```python
from build123d import *

# Parameters (mm, degrees)
SKETCH1_W           = 17.9
SKETCH1_H           = 14
BOSS_EXTRUDE1_DEPTH = 6
SKETCH2_R           = 1.75
CUT_EXTRUDE1_DEPTH  = 15
CUT_EXTRUDE2_DEPTH  = 6
CHAMFER1_SIZE       = 0.25


with BuildPart() as part:
    # Sketch1 → Boss-Extrude1 (new body)
    with BuildSketch(Plane.XY):
        with Locations((0, 7)):
            Rectangle(SKETCH1_W, SKETCH1_H)
    extrude(amount=BOSS_EXTRUDE1_DEPTH)

    # Sketch2 → Cut-Extrude1 (cut, through all)
    with BuildSketch(Plane(origin=(0, 14, 0), x_dir=(1, 0, 0), z_dir=(0, 1, 0))):
        with Locations((0, -3)):
            Circle(SKETCH2_R)
    extrude(amount=-CUT_EXTRUDE1_DEPTH, mode=Mode.SUBTRACT)

    # Sketch3 → Cut-Extrude2 (cut)
    with BuildSketch(Plane.XY.offset(6)):
        Polygon((5, 14), (5, 2), (5.7, 2), (5.7, 2.2), (6.6, 3.1), (5.7, 4), (5.7, 4.2), (6.6, 5.1), (5.7, 6), (5.7, 6.2), (6.6, 7.1), (5.7, 8), (5.7, 8.2), (6.6, 9.1), (5.7, 10), (5.7, 10.2), (6.6, 11.1), (5.7, 12), (5.7, 12.2), (6.6, 13.1), (5.7, 14), align=None)
        Polygon((-5.7, 2.2), (-5.7, 2), (-5, 2), (-5, 14), (-5.7, 14), (-6.6, 13.1), (-5.7, 12.2), (-5.7, 12), (-6.6, 11.1), (-5.7, 10.2), (-5.7, 10), (-6.6, 9.1), (-5.7, 8.2), (-5.7, 8), (-6.6, 7.1), (-5.7, 6.2), (-5.7, 6), (-6.6, 5.1), (-5.7, 4.2), (-5.7, 4), (-6.6, 3.1), align=None)
    extrude(amount=-CUT_EXTRUDE2_DEPTH, mode=Mode.SUBTRACT)

    # Chamfer1
    chamfer1_edges = [part.edges().sort_by_distance(p)[0] for p in [
        (8.95, 7, 6),
        (0, 14, 0),
        (-7.325, 14, 0),
        (-8.95, 7, 6),
        (7.325, 14, 0),
        (8.95, 7, 0),
        (0, 0, 0),
        (-8.95, 7, 0),
        (0, 0, 6),
    ]]
    chamfer(chamfer1_edges, length=CHAMFER1_SIZE)


solid = part.part
```
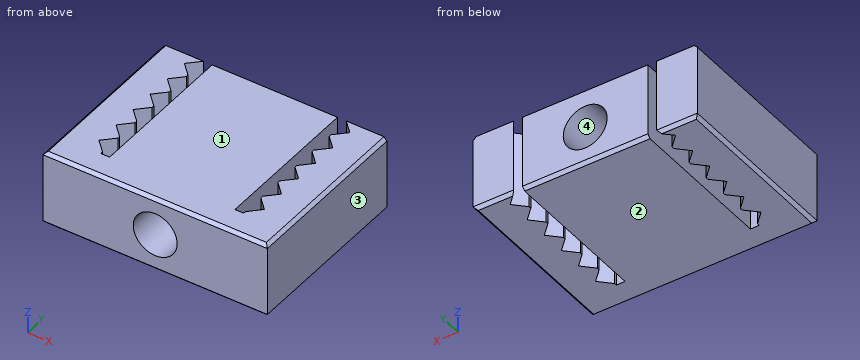
Input: part model. Units: mm. Frame: model coordinates. Face numbers are marked on the shaded views. Round coordinates to 2 decimals unless told otherwise and drop trailing zeros. Write each loop counter-clockwise with the first axis right and the second up, starting at its lowest first coordinate (ties: lowest second). Pieces come first, ordered by that corner, then holes. Notation, with made-up numbers: M 84.5,54.5 L 131.5,54.5 A15 cw 131.5,74.5 Z; hole C 68.5,1 d4. An arc over 180 degrees is marked long. Write each question's results on one line, items separated by ' | '.
Q1. Draft query along Z for the marked faces 1, 2, 3 and 4. Return one class per face: released by +Z, released by -Z, zero draft, split by the parting line, or undercut.
Results:
face 1: released by +Z | face 2: released by -Z | face 3: zero draft | face 4: undercut
Q2. Pin query (flat end, axial travel): P1, Ø2, axis at x = 0, z = 3, coming from the -Y side. Return the tip coordinate at first contact, or that it passes through.
Results:
P1: passes through
Q3. Section query A-A (y = 7.5). Return loops of the section in (x, z).
Results:
outline: M -8.95,0.25 L -8.7,0 L -6.2,0 L -6.2,6 L -8.7,6 L -8.95,5.75 Z; M -5,0 L 5,0 L 5,6 L -5,6 Z; M 6.2,0 L 8.7,0 L 8.95,0.25 L 8.95,5.75 L 8.7,6 L 6.2,6 Z; hole C 0,3 d3.5
Q4. Section query B-B (x = 0). Return loops of the section in (y, z), and give its area (3 significant figures).
Results:
outline: M 0,0.25 L 0.25,0 L 13.75,0 L 14,0.25 L 14,1.25 L 0,1.25 Z; M 0,4.75 L 14,4.75 L 14,6 L 0.25,6 L 0,5.75 Z | area: 34.9 mm^2
Q5. Line query: line 1 along X through (y, z) = (6.5, 2.25); line 2 along X through (y, z) = (9.5, 3); line 3 along X through (y, z) = (11.5, 0.75). Output: solid intervals per line, ascending.
Results:
line 1: x = -8.95 to -6, -5 to -1.58, 1.58 to 5, 6 to 8.95 | line 2: x = -8.95 to -6.2, -5 to -1.75, 1.75 to 5, 6.2 to 8.95 | line 3: x = -8.95 to -6.2, -5 to 5, 6.2 to 8.95
Q6. Section query C-C (y = 1.5). Return loops of the section in (x, z).
Results:
outline: M -8.95,0.25 L -8.7,0 L 8.7,0 L 8.95,0.25 L 8.95,5.75 L 8.7,6 L -8.7,6 L -8.95,5.75 Z; hole C 0,3 d3.5
